Design review of the part built by this model. Coordinates are the model's own, in mm. A direction names the side the tool comes from. Give positions to 0.01 mm unless a question says otherwise; leave off trailing zeros. Order: outer loops, then holes, each group sorted by start corner. A loop starts at its lowest first (then second) coordinate and runs counter-clockwise, first axis right, second up. Notation, with made-up numbers: (-2.5, 17) -> (41.5, 17) arc R12 cw to (41.5, 29) -> close; hole circle Ø7 at (-15, 32). An arc over 180 degrees is marked (long way). One line per item, written item: value. Start each with the question number.
1) Consider section C-C (x = -2.5). State the section outline as (y, z) points, plus the area to 3 significant figures.
2) The part is to be moulded in two halves that separate along Y. For faces 1 (the face through (0, 0, -3)), 2 (the face through (11.85, -1.51, 13.03)), 3 (the face through (-2.825, -1.479, -9.464)), say which applies: released by +Y, released by -Y, zero draft, split by the parting line, or undercut.
3) For pin 1 (1 mm diameter, centred on y = -1, z = -8.5, fed in from +X), flat-tipped, find the tip position at first contact; note if it passes through.
4) Consider section A-A (z = 2). State the section outline as (x, y) points.
5) Consider section D-D (z = 11.5). State the section outline as (x, y) points, plus the area to 3 significant figures.
6) Tool access review of faces 4 (the face through (12.5, -0.5, 9.9)), 5 (the face through (11.5, -1, -5)), 6 (the face through (-2, -1, 10)): name each direction out of +Z, -Z, +X, -X, +Y, -Y from which nothing blocks a thin tool from reaching the whole face with its end or side.
7) Wall thickness on line 1 along Z through (x, y) = (-2.5, -1.9); line 2 along X through (y, z) = (-2.05, -10.5); line 3 along Z through (x, y) = (-7.5, -2.3): over which ranges is each line inside the solid? List them lowest first. Write a range as from..to.
8) Consider section B-B (y = -0.4). State the section outline as (x, z) points, plus the area to 3 significant figures.
from build123d import *

# Parameters (mm, degrees)
F0_R     = 1.5
F1_DEPTH = 3
F4_W     = 0.5
F4_H     = 7.027182
F5_DEPTH = 0.5


with BuildPart() as f1:
    # F0 (on Front) → F1 (new body)
    with BuildSketch(Plane.XZ):
        Polygon((12.5, 5), (12.5, 15), (10.5, 15), (7.5, 10), (-12.5, 10), (-12.5, -15), (11.5, -15), (11.5, 5), align=None)
        with Locations((-2.5, -8)):
            Circle(F0_R, mode=Mode.SUBTRACT)
        with Locations((-2.5, 2)):
            Circle(F0_R, mode=Mode.SUBTRACT)
    extrude(amount=F1_DEPTH)

    # F2 (on face) → F3 (revolve, cut)
    with BuildSketch(Plane.YZ.offset(12.5)):
        Polygon((-0.85, 15.881686), (-1.5, 15.881686), (-1.5, 10), (-1.2, 10), (-0.85, 11), align=None)
    revolve(axis=Axis((12.5, -1.5, 3.419226), (0, 0, -1)), mode=Mode.SUBTRACT)

    # F4 (on face) → F5 (cut)
    with BuildSketch(Plane.YZ.offset(12.5)):
        with Locations((-1.5, 7.433284)):
            Rectangle(F4_W, F4_H)
    extrude(amount=-F5_DEPTH, mode=Mode.SUBTRACT)


solid = f1.part
Checked values:
1. outline: (-3, -15) -> (0, -15) -> (0, -9.5) -> (-3, -9.5) -> close; (-3, -6.5) -> (0, -6.5) -> (0, 0.5) -> (-3, 0.5) -> close; (-3, 3.5) -> (0, 3.5) -> (0, 10) -> (-3, 10) -> close
1. area: 57.0 mm^2
2. face 1: released by +Y
2. face 2: undercut
2. face 3: zero draft
3. pin 1: stops at x = 11.5
4. outline: (-12.5, -3) -> (-4, -3) -> (-4, 0) -> (-12.5, 0) -> close; (-1, -3) -> (11.5, -3) -> (11.5, 0) -> (-1, 0) -> close
5. outline: (8.4, -3) -> (12.5, -3) -> (12.5, -2.15) arc R0.65 cw to (12.5, -0.85) -> (12.5, 0) -> (8.4, 0) -> close
5. area: 11.6 mm^2
6. face 4: +Z, -Z, +X, +Y, -Y
6. face 5: -Z, +X, +Y, -Y
6. face 6: +Z, -X, +Y, -Y
7. line 1: z = -15..-9.5, -6.5..0.5, 3.5..10
7. line 2: x = -12.5..11.5
7. line 3: z = -15..10
8. outline: (-12.5, -15) -> (11.5, -15) -> (11.5, 5) -> (12.5, 5) -> (12.5, 15) -> (10.5, 15) -> (7.5, 10) -> (-12.5, 10) -> close; hole circle Ø3 at (-2.5, -8); hole circle Ø3 at (-2.5, 2)
8. area: 608 mm^2
